Design review of the part shown in the three views and the two pictorial views. Dimensions are in mm from the part's minimum x, y and z. Give positions to 0.01 mm unless a question says otherwise; leave off trailing zeros. Order: outer loops, then holes, each group sorted by start corner. A loop starts at its lowest first (then second) coordinate and runs counter-clockwise, first axis right, second up.
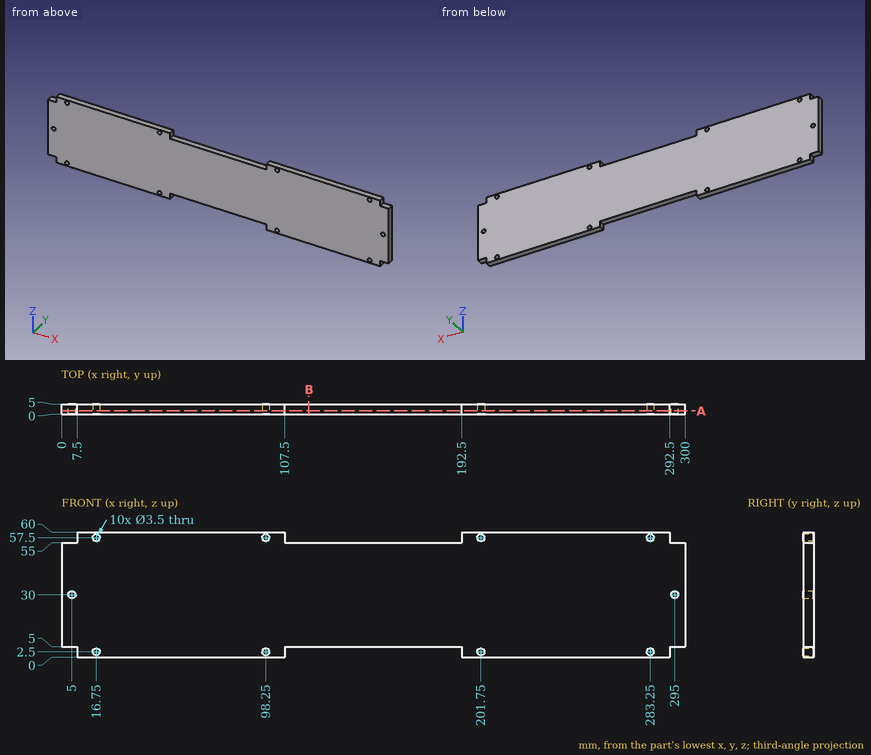
1) To check wall thickness, follow line 1 (X direction, y = 3.3, z = 2.5); line 2 (Z direction, x = 16.75, y = 2.3); line 3 (X direction, y = 2.5, z = 30). State the ranges of each line that lie inside material, in increasing order.
Answer sheet:
line 1: x = 7.5 to 15, 18.5 to 96.5, 100 to 107.5, 192.5 to 200, 203.5 to 281.5, 285 to 292.5
line 2: z = 0 to 0.75, 4.25 to 55.75, 59.25 to 60
line 3: x = 0 to 3.25, 6.75 to 293.25, 296.75 to 300
2) Clearance check with flat-ended pins moving along their axes: pin 1 (2.5 mm diameter, centred on y = 1.5, z = 2, fed in from +X); pin 2 (1.5 mm diameter, centred on x = 140, y = 3.5, fed in from -Z). State where each tip first meets the part, or that it passes through.
Answer sheet:
pin 1: stops at x = 292.5
pin 2: stops at z = 5
3) We need section B-B on x = 119. Give the boundary of the cut face in (y, z), then the cut area to 3 significant figures.
Answer sheet:
outline: (0, 5) - (5, 5) - (5, 55) - (0, 55) - close
area: 250 mm2
4) We need section A-A on y = 1.65. Count the separate pieces of the cut face and the enclosed holes in it, then the cut area to 3 significant figures.
Answer sheet:
separate pieces: 1
enclosed holes: 10
area: 16,900 mm2
